Input: part model. Units: mm. Frame: model coordinates. Face numbers are marked on the shaded views. A direction names the side the tool comes from. Coordinates: 2 decimals unless noted, no trailing zeros. Loops run counter-clockwise (first coordinate to the right, second up) from the corner with the lowest first, then second, coordinate; pieces in that order, holes last. Notation, with made-up numbers: (20, -29) -> (57, -29) arc R21 cw to (57, -24) -> close; hole circle Ø4 at (-24, 88). An arc over 180 degrees is marked (long way). Answer as a JSON object with one key per item and string values.
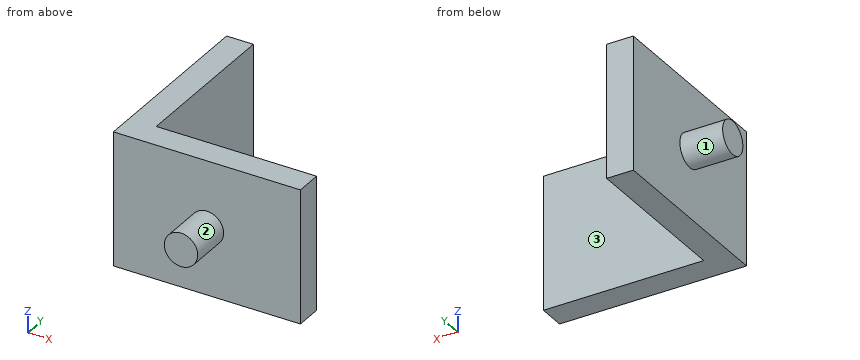
from build123d import *

# Parameters (mm, degrees)
BOSS_EXTRUDE1_DEPTH = 20
SKETCH5_R           = 2.5
BOSS_EXTRUDE6_DEPTH = 6.4
SKETCH6_R           = 2.5
BOSS_EXTRUDE7_DEPTH = 6.4


with BuildPart() as part:
    # Sketch1 → Boss-Extrude1 (new body)
    with BuildSketch(Plane.XY):
        Polygon((0, 0), (0, 28), (4, 28), (4, 4), (28, 4), (28, 0), align=None)
    extrude(amount=BOSS_EXTRUDE1_DEPTH)

    # Sketch5 → Boss-Extrude6 (add)
    with BuildSketch(Plane.ZY):
        with Locations((10, 14)):
            Circle(SKETCH5_R)
    extrude(amount=BOSS_EXTRUDE6_DEPTH)

    # Sketch6 → Boss-Extrude7 (add)
    with BuildSketch(Plane.XZ):
        with Locations((14, 10)):
            Circle(SKETCH6_R)
    extrude(amount=BOSS_EXTRUDE7_DEPTH)


solid = part.part
1. Section query C-C (z = 5.25). Return loops of the section in (x, y).
Reply:
{"outline": "(0, 0) -> (28, 0) -> (28, 4) -> (4, 4) -> (4, 28) -> (0, 28) -> close"}
2. Section query A-A (y = 16). Return loops of the section in (x, z).
Reply:
{"outline": "(-6.4, 8.5) -> (0, 8.5) -> (0, 0) -> (4, 0) -> (4, 20) -> (0, 20) -> (0, 11.5) -> (-6.4, 11.5) -> close"}
3. Pin query (flat end, axial travel): P1, Ø4, axis at y = 24.5, z = 4.5, coming from the +X side; P2, Ø10, axis at x = 16.5, z = 14, coming from the +Y side; P3, Ø6, axis at x = -2.5, z = 9, coming from the -Y side. Return the tip coordinate at first contact, or that it passes through.
Reply:
{"P1": "stops at x = 4", "P2": "stops at y = 4", "P3": "stops at y = 0"}
4. Section query B-B (x = 14). Return loops of the section in (y, z).
Reply:
{"outline": "(-6.4, 7.5) -> (0, 7.5) -> (0, 0) -> (4, 0) -> (4, 20) -> (0, 20) -> (0, 12.5) -> (-6.4, 12.5) -> close"}
5. Section query D-D (z = 10). Return loops of the section in (x, y), plus the area to 3 significant figures.
Reply:
{"outline": "(-6.4, 11.5) -> (0, 11.5) -> (0, 0) -> (11.5, 0) -> (11.5, -6.4) -> (16.5, -6.4) -> (16.5, 0) -> (28, 0) -> (28, 4) -> (4, 4) -> (4, 28) -> (0, 28) -> (0, 16.5) -> (-6.4, 16.5) -> close", "area": "272 mm2"}
6. Access query for the marked faces 1, 2 and 3. Directions: +Z, -Z, +X, -X, +Y, -Y. A direction counts if a zero-diameter tool reaches every point of the face in a straight line with its end or side. Return the directions, or none.
Reply:
{"face 1": "-X", "face 2": "-Y", "face 3": "+Z, -Z, +X, +Y"}
7. Line query: line 1 along X through (y, z) = (15, 7); line 2 along Y through (x, z) = (1, 9). Output: solid intervals per line, ascending.
Reply:
{"line 1": "x = 0 to 4", "line 2": "y = 0 to 28"}
